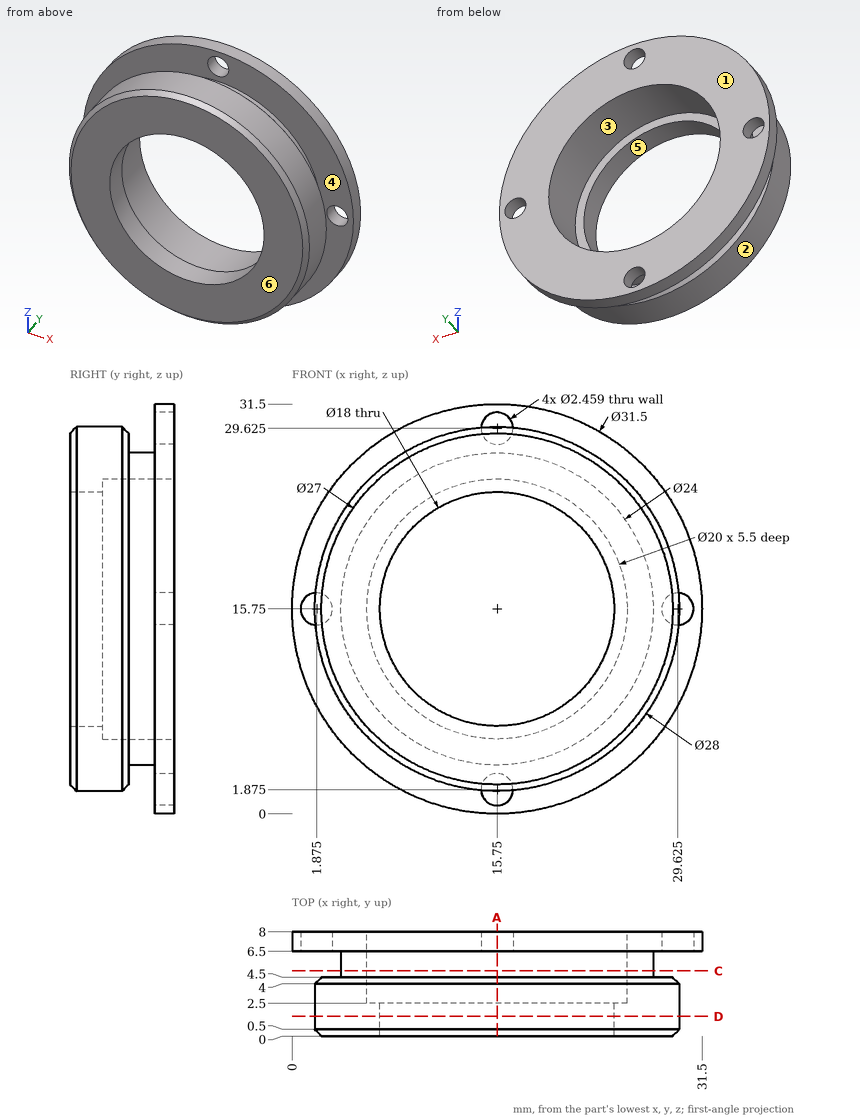
Geometry: see drawing. Coordinates: mm, zero at the bounding-box minimum. A direction names the side the tool comes from. Coordinates: 2 decimals unless noted, no trailing zeros. Loops run counter-clockwise (first coordinate to the right, second up) from the corner with the lowest first, then second, coordinate; pieces in that order, holes last.
Q1. Contact query for flat-ended pins moving along their axis: pin 1 (1.5 mm diameter, centred on y = 1, z = 27.5, fed in from +X); pin 2 (2 mm diameter, centred on x = 15.75, z = 1.875, fed in from +Y). Output: stop coordinate, or through.
Q2. Draft query along Y for the marked faces 4, 5 and 6. Return one class per face: +Y half, -Y half, draft (parallel to the pull), parting line (faces both ways), or undercut.
Q3. Material intervals for line 1 (X direction, y = 6.95, z = 15.75); line 2 (X direction, y = 1.2, z = 15.75), sorted ascending.
Q4. Cut plane D-D (y = 1.5). Output: boundary loops of the cut face in (x, z), then the cut area to 3 significant figures.
Q5. Set-up query: the marked faces 1, 2 and 3. Return all of +Z, -Z, +X, -X, +Y, -Y with unobstructed straight access to the full face (end or side cutting, diameter ignored); none if empty.
Q6. Cut plane A-A (x = 15.75). Give the number of separate pieces and of enclosed holes in the cut face, then the cut area to 3 significant figures.
Q7. Cut plane C-C (y = 5). Output: boundary loops of the cut face in (x, z), then the cut area to 3 significant figures.
Working result:
1. pin 1: stops at x = 24.41
1. pin 2: stops at y = 4.5
2. face 4: undercut
2. face 5: draft
2. face 6: -Y half
3. line 1: x = 0 to 0.65, 3.1 to 5.75, 25.75 to 28.4, 30.85 to 31.5
3. line 2: x = 1.75 to 6.75, 24.75 to 29.75
4. outline: circle Ø28 at (15.75, 15.75); hole circle Ø18 at (15.75, 15.75)
4. area: 361 mm2
5. face 1: +Z, -Z, +X, -X, +Y
5. face 2: -Y
5. face 3: +Y
6. separate pieces: 4
6. enclosed holes: 0
6. area: 58.4 mm2
7. outline: circle Ø24 at (15.75, 15.75); hole circle Ø20 at (15.75, 15.75)
7. area: 138 mm2
